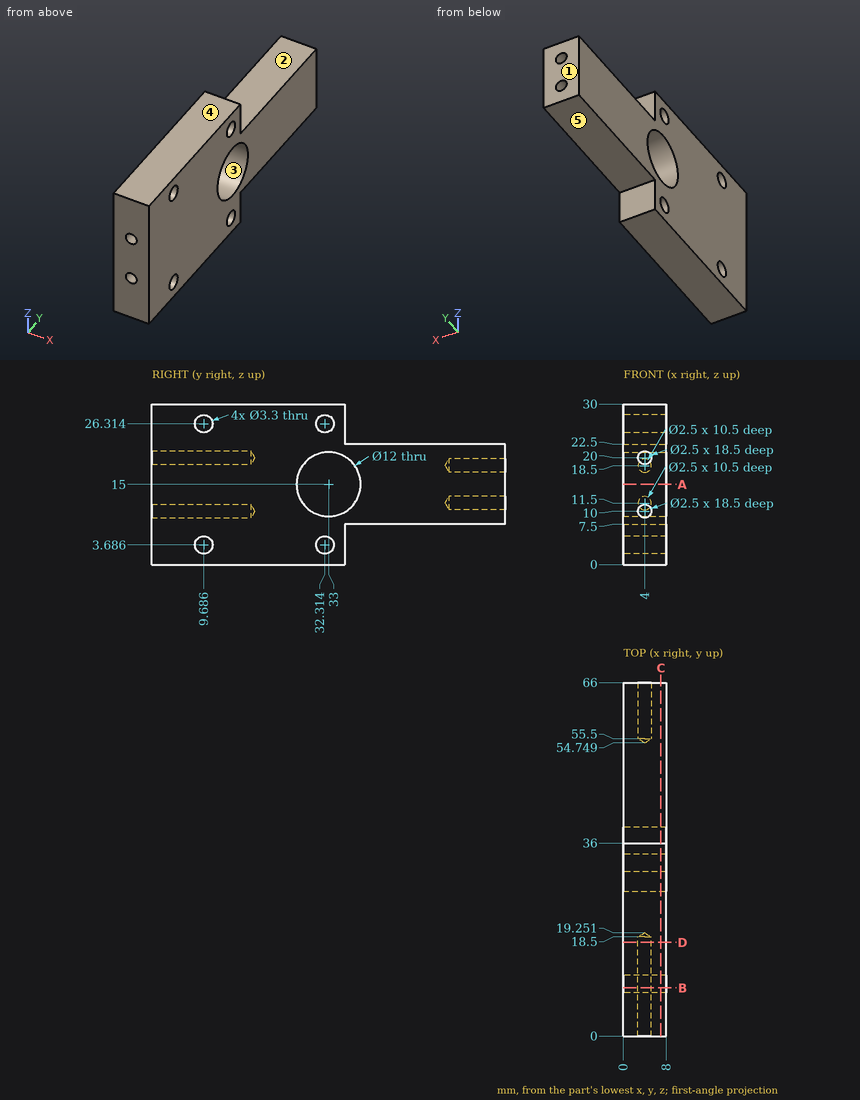
Print and shaded views of the part. All mm, measured from the part's lowest x, y and z. A direction names the side the tool comes from. Round coordinates to 2 decimals unless told otherwise and drop trailing zeros. Write each loop counter-clockwise with the first axis right and the second up, starting at its lowest first coordinate (ties: lowest second). Pieces come first, ordered by that corner, then holes. Notation, with made-up numbers: (84, -15.75) -> (88, -15.75) arc R34 cw to (88, 22.25) -> close; hole circle Ø2 at (85.5, 21). An arc over 180 degrees is marked (long way). Return JSON: item names as keys, results as strings. Group by question number.
Q1. Pin check, flat tips, straight feed: pin 1 (2 mm diameter, centred on y = 32.31, z = 3.69, fed in from -X); pin 2 (2 mm diameter, centred on x = 4, z = 10, fed in from -Y); pin 3 (1.5 mm diameter, centred on x = 7, y = 51, fed in from -Z); pin 4 (2 mm diameter, centred on x = 2.5, z = 27, fed in from +Y). Stop position of each tip, or through.
Q2. Probe L1, parallel to Z at x = 4, y = 7.75; L2, parallel to Z at x = 4, y = 63; L3, parallel to Y at x = 7, z = 25.75 (1 decimal). List the from-to ranges inside material, lowest first. Write a range as [from, to].
Q3. Mould opens along Z. For the marked faces 1, 2 and 3 say: pulls with the +Z half, pulls with the -Z half, needs draft (parallel to the pull), parting line crosses it, or undercut.
Q4. Saw through at A-A on z = 15. Write the cut outline in (x, y), plus the area to 3 significant figures.
Q5. Saw through at B-B on y = 9. Write the cut outline in (x, z), plus the area to 3 significant figures.
Q6. Saw through at D-D on y = 17.5. Write the cut outline in (x, z).
Q7. Which spindle directions (+Z, -Z, +X, -X, +Y, -Y) get a long thin tool onto all of the face, cutting with end or side? Do the marked faces 4 and 5. Say none if no direction does.
Q8. Saw through at C-C on x = 7. Write the cut outline in (y, z).
Answer:
{
 "1": {"pin 1": "through", "pin 2": "y = 18.65", "pin 3": "z = 7.5", "pin 4": "y = 36"},
 "2": {"L1": "[0, 8.75], [11.25, 18.75], [21.25, 30]", "L2": "[7.5, 10.25], [12.75, 17.25], [19.75, 22.5]", "L3": "[0, 8.1], [11.2, 30.8], [33.9, 36]"},
 "3": {"face 1": "needs draft", "face 2": "pulls with the +Z half", "face 3": "undercut"},
 "4": {"outline": "(0, 0) -> (8, 0) -> (8, 27) -> (0, 27) -> close; (0, 39) -> (8, 39) -> (8, 66) -> (0, 66) -> close", "area": "432 mm2"},
 "5": {"outline": "(0, 0) -> (8, 0) -> (8, 2.19) -> (0, 2.19) -> close; (0, 5.19) -> (8, 5.19) -> (8, 24.81) -> (0, 24.81) -> close; (0, 27.81) -> (8, 27.81) -> (8, 30) -> (0, 30) -> close; hole circle Ø2.5 at (4, 10); hole circle Ø2.5 at (4, 20)", "area": "182 mm2"},
 "6": {"outline": "(0, 0) -> (8, 0) -> (8, 30) -> (0, 30) -> close; hole circle Ø2.5 at (4, 10); hole circle Ø2.5 at (4, 20)"},
 "7": {"face 4": "+Z, +X, -X, +Y, -Y", "face 5": "-Z, +X, -X, +Y"},
 "8": {"outline": "(0, 0) -> (36, 0) -> (36, 7.5) -> (66, 7.5) -> (66, 22.5) -> (36, 22.5) -> (36, 30) -> (0, 30) -> close; hole circle Ø3.3 at (9.69, 3.69); hole circle Ø3.3 at (9.69, 26.31); hole circle Ø12 at (33, 15); hole circle Ø3.3 at (32.31, 3.69); hole circle Ø3.3 at (32.31, 26.31)"}
}
